Here's how the part is built. I have some questions about the finished solid (model axes, mm). Coordinates: 2 decimals unless noted, no trailing zeros. Order: outer loops, then holes, each group sorted by start corner. A loop starts at its lowest first (then second) coordinate and runs counter-clockwise, first axis right, second up.
```python
from build123d import *

# Parameters (mm, degrees)
SKETCH1_W               = 40
SKETCH1_H               = 20
BOSS_EXTRUDE1_DEPTH     = 10
CUT_EXTRUDE1_DEPTH      = 46.82575695
CUT_EXTRUDE1_DEPTH_BACK = 46.82575695
SKETCH2_R               = 4


with BuildPart() as part:
    # Sketch1 → Boss-Extrude1 (new, symmetric)
    with BuildSketch(Plane.XY):
        with Locations((20, 10)):
            Rectangle(SKETCH1_W, SKETCH1_H)
    extrude(amount=BOSS_EXTRUDE1_DEPTH, both=True)

    # Sketch2 → Cut-Extrude1 (cut, two sides: drawn at the far end of the back side and taken through both)
    with BuildSketch(Plane.XY.offset(-CUT_EXTRUDE1_DEPTH_BACK)):
        with Locations((20, 10)):
            Circle(SKETCH2_R)
    extrude(amount=CUT_EXTRUDE1_DEPTH + CUT_EXTRUDE1_DEPTH_BACK, mode=Mode.SUBTRACT)


solid = part.part
```
Q1. I need wall thicknesses on L1, parallel to Y at x = 20, z = -5; L2, parallel to X at y = 10, z = 3; L3, parallel to Y at x = 17.5, z = 0.5. Which ranges of each line are inside material? Lowest first, please.
Q2. We'd pull the mould along Y, two halves only. Please class faces 1 (the cylindrical face through (19.479, 13.966, -0.14)), 2 (the flat face through (40, 10, 0)), 3 (the flat face through (20, 0, 0)), 4 (the flat face through (20, 20, 0)): pulls with the +Y half, pulls with the -Y half, needs draft (parallel to the pull), parting line crosses it, or undercut.
Q3. Will these pins go through, and if not, where does the flat tip stop? pin 1 (1.5 mm diameter, centred on x = 31.5, z = -0.5, fed in from -Y); pin 2 (7 mm diameter, centred on x = 20, y = 10, fed in from -Z).
Q4. If we section it at C-C on z = 2.25: Write out the boundary of the cut face in (x, y).
Q5. If we section it at B-B on x = 20: Write out the boundary of the cut face in (y, z).
Q6. If we section it at A-A on y = 10: Write out the boundary of the cut face in (x, z), then the cut area to 3 significant figures.
Reply:
1. L1: y = 0 to 6, 14 to 20
1. L2: x = 0 to 16, 24 to 40
1. L3: y = 0 to 6.88, 13.12 to 20
2. face 1: undercut
2. face 2: needs draft
2. face 3: pulls with the -Y half
2. face 4: pulls with the +Y half
3. pin 1: stops at y = 0
3. pin 2: passes through
4. outline: (0, 0) - (40, 0) - (40, 20) - (0, 20) - close; hole circle Ø8 at (20, 10)
5. outline: (0, -10) - (6, -10) - (6, 10) - (0, 10) - close; (14, -10) - (20, -10) - (20, 10) - (14, 10) - close
6. outline: (0, -10) - (16, -10) - (16, 10) - (0, 10) - close; (24, -10) - (40, -10) - (40, 10) - (24, 10) - close
6. area: 640 mm2
